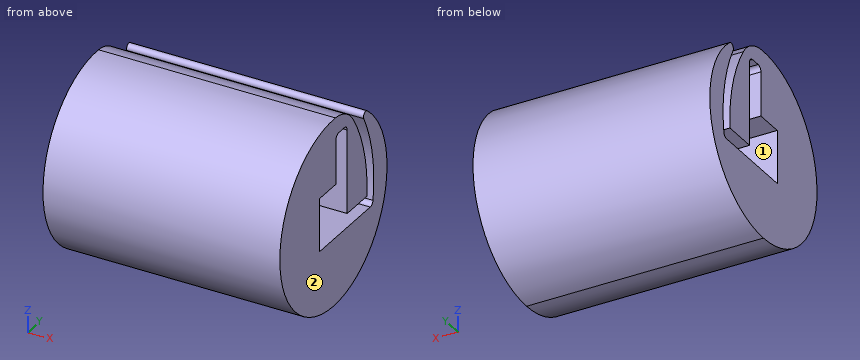
```python
from build123d import *

# Parameters (mm, degrees)
BOSS_EXTRUDE2_DEPTH = 6
FILLET1_R           = 0.25
FILLET2_R           = 2
FILLET3_R           = 0.2


with BuildPart() as part:
    # Sketch1 → Boss-Extrude2 (new, symmetric)
    with BuildSketch(Plane(origin=(0, 0, 0), x_dir=(0, 0, -1), z_dir=(1, 0, 0))):
        with BuildLine():
            Line((-1.35, -1.225), (-1.35, 0.225))
            Line((-1.35, 0.225), (-3.85, 0.225))
            Line((-3.85, 0.225), (-3.85, 1.225))
            Line((-3.85, 1.225), (-1.35, 1.225))
            Line((-1.35, 1.225), (0.648540494, 1.225))
            Line((0.648540494, 1.225), (0.648540494, 2.975))
            ThreePointArc((0.648540494, 2.975), (-2.137325495, 2.599646629), (-4.589321845, 1.225))
            ThreePointArc((-4.589321845, 1.225), (-0.617746402, -4.709659158), (4.75, 0))
            ThreePointArc((4.75, 0), (1.146387884, 4.609587272), (-4.19665045, 2.225))
            ThreePointArc((-4.19665045, 2.225), (-1.546369522, 3.395986963), (1.35, 3.475))
            Line((1.35, 3.475), (1.35, 1.225))
            Line((1.35, 1.225), (1.35, -1.225))
            Line((1.35, -1.225), (-1.35, -1.225))
        make_face()
    extrude(amount=BOSS_EXTRUDE2_DEPTH, both=True)

    # Fillet1
    fillet1_edges = [part.edges().sort_by_distance(p)[0] for p in [
        (0, 1.225, 3.85),
        (0, 0.225, 3.85),
        (0, 3.475, -1.35),
    ]]
    fillet(fillet1_edges, radius=FILLET1_R)

    # Fillet2
    fillet2_edges = [part.edges().sort_by_distance(p)[0] for p in [
        (0, 1.225, 4.589321845),
    ]]
    fillet(fillet2_edges, radius=FILLET2_R)

    # Fillet3
    fillet3_edges = [part.edges().sort_by_distance(p)[0] for p in [
        (0, 2.225, 4.19665045),
    ]]
    fillet(fillet3_edges, radius=FILLET3_R)


solid = part.part
```
Work out the finished part from the listing and answer in its coordinate system (mm). Face numbers are marked on the shaded views. A direction names the side the tool comes from. Coordinates: 2 decimals unless noted, no trailing zeros. Order: outer loops, then holes, each group sorted by start corner. A loop starts at its lowest first (then second) coordinate and runs counter-clockwise, first axis right, second up. Notation, with made-up numbers: (-24, 9) - (22, 9) arc R29 ccw to (22, 45) - close; hole circle Ø10 at (-0.75, -30). An arc over 180 degrees is marked (long way). Answer as a JSON object with one key per item and string values.
1. Find section C-C on z = -0.5. Determine the outline of the cut face in (x, y) (3 decimals).
Output values:
{"outline": "(-6, -4.724) - (6, -4.724) - (6, -1.225) - (-6, -1.225) - close; (-6, 1.225) - (6, 1.225) - (6, 2.982) - (-6, 2.982) - close; (-6, 3.569) - (6, 3.569) - (6, 4.724) - (-6, 4.724) - close"}
2. Each of these flat-tipped pins is pushed along its axis until it touches: P1, Ø1, axis at x = 0.5, z = -1, coming from the +Y side; P2, Ø2.5, axis at x = 3, z = 3, coming from the +Y side; P3, Ø0.9, axis at x = 0.5, y = 2, coming from the -Z side. Where does it stop, or does it pass through?
Output values:
{"P1": "stops at y = 4.72", "P2": "stops at y = 4.42", "P3": "stops at z = -4.49"}
3. A tool of negligible diameter and unlimited length cuts with its end or side. For the marked faces 1 and 2, from which of +Z, -Z, +X, -X, +Y, -Y can it reach the whole face along a straight path? Write none if from no direction.
Output values:
{"face 1": "+X, -X", "face 2": "+Z, -Z, +X, +Y, -Y"}
4. Find section A-A on z = 2. Determine the outline of the cut face in (x, y) (3 decimals), plus the area to 3 significant figures.
Output values:
{"outline": "(-6, -4.308) - (6, -4.308) - (6, 0.225) - (-6, 0.225) - close; (-6, 1.225) - (6, 1.225) - (6, 2.644) - (-6, 2.644) - close; (-6, 3.279) - (6, 3.279) - (6, 4.308) - (-6, 4.308) - close", "area": "83.8 mm²"}
5. Consider line 1 (Y direction, x = -3.5, z = 0) (3 decimals); line 2 (Z direction, x = 4.5, y = 0); line 3 (Y direction, x = 3, z = 3.5) (3 decimals). Determine where each line is inside the solid, lowest interval first.
Output values:
{"line 1": "y = -4.75 to -1.225, 1.225 to 2.982, 3.579 to 4.75", "line 2": "z = -4.75 to -1.35, 1.35 to 4.75", "line 3": "y = -3.211 to 0.225, 1.225 to 1.988, 2.67 to 3.211"}
6. Find section B-B on y = 2.5. Determine the outline of the cut face in (x, z).
Output values:
{"outline": "(-6, -4.04) - (6, -4.04) - (6, -1.35) - (-6, -1.35) - close; (-6, -0.65) - (6, -0.65) - (6, 2.42) - (-6, 2.42) - close"}
